Geometry: see drawing. Coordinates: mm, zero at the bounding-box minimum. A direction names the side the tool comes from. Round coordinates to 2 decimals unless told otherwise and drop trailing zeros. Order: outer loops, then holes, each group sorted by start corner. A loop starts at its lowest first (then second) coordinate and runs counter-clockwise, first axis right, second up. Notation, with made-up numbers: (36.25, 36) -> (78.25, 36) arc R7 ccw to (78.25, 42) -> close; hole circle Ø11 at (87.5, 47.25). An arc over 180 degrees is marked (long way). Use a Markdown table: item, result.
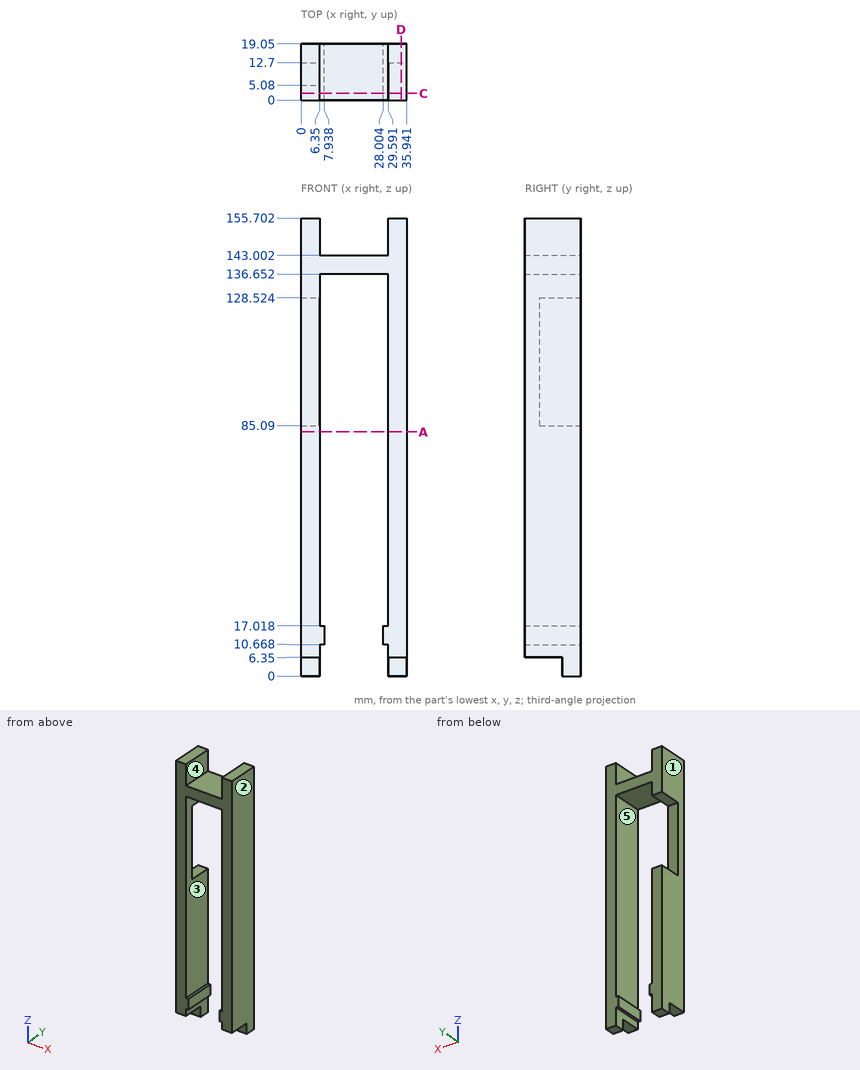
1) Ray query, probe 1 along Z at (x, y) = (28.5, 14.75); probe 2 along X at (y, z) = (12, 33); probe 3 along Z at (x, y) = (13, 6). Return the intervals inside material, ascending.
Answer key:
| item | result |
|---|---|
| probe 1 | z = 10.67 to 17.02, 136.65 to 143 |
| probe 2 | x = 0 to 6.35, 29.59 to 35.94 |
| probe 3 | z = 136.65 to 143 |
2) Cut plane D-D on x = 34. Return loops of the section in (y, z).
Answer key:
| item | result |
|---|---|
| outline | (0, 6.35) -> (12.7, 6.35) -> (12.7, 0) -> (19.05, 0) -> (19.05, 155.7) -> (0, 155.7) -> close |
3) Cut plane C-C on y = 2.25. Return loops of the section in (x, z).
Answer key:
| item | result |
|---|---|
| outline | (0, 6.35) -> (6.35, 6.35) -> (6.35, 10.67) -> (7.94, 10.67) -> (7.94, 17.02) -> (6.35, 17.02) -> (6.35, 136.65) -> (29.59, 136.65) -> (29.59, 17.02) -> (28, 17.02) -> (28, 10.67) -> (29.59, 10.67) -> (29.59, 6.35) -> (35.94, 6.35) -> (35.94, 155.7) -> (29.59, 155.7) -> (29.59, 143) -> (6.35, 143) -> (6.35, 155.7) -> (0, 155.7) -> close |
4) Draft query along X for the marked faces 1, 2 and 3. Return one class per face: released by +X, released by -X, zero draft, split by the parting line, or undercut.
Answer key:
| item | result |
|---|---|
| face 1 | released by -X |
| face 2 | released by +X |
| face 3 | undercut |
5) Cut plane A-A on z = 83. Return loops of the section in (x, y), and give its area (3 significant figures).
Answer key:
| item | result |
|---|---|
| outline | (0, 0) -> (6.35, 0) -> (6.35, 19.05) -> (0, 19.05) -> close; (29.59, 0) -> (35.94, 0) -> (35.94, 19.05) -> (29.59, 19.05) -> close |
| area | 242 mm^2 |
6) Contact query for flat-ended pins moving along their axis: P1, Ø0.8, axis at x = 7.5, y = 9, coming from the -Z side; P2, Ø9.5, axis at y = 11.5, z = 61.5, coming from the -X side; P3, Ø7, axis at x = 3, z = 2.5, coming from the -Y side; P4, Ø3, axis at x = 34, y = 4.5, coming from the -Z side. Output: stop coordinate, or through.
Answer key:
| item | result |
|---|---|
| P1 | stops at z = 10.67 |
| P2 | stops at x = 0 |
| P3 | stops at y = 12.7 |
| P4 | stops at z = 6.35 |
7) Set-up query: the marked faces 4 and 5. Return all of +Z, -Z, +X, -X, +Y, -Y with unobstructed straight access to the full face (end or side cutting, diameter ignored); none if empty.
Answer key:
| item | result |
|---|---|
| face 4 | +Z, +Y, -Y |
| face 5 | +Y, -Y |
